Could you check a few things on this drawing? It's one solid part, dimensions in mm from its lowest x, y, z. A direction names the side the tool comes from. Give positions to 0.01 mm unless a question says otherwise; leave off trailing zeros. Order: outer loops, then holes, each group sorted by start corner. A loop starts at its lowest first (then second) coordinate and runs counter-clockwise, first axis right, second up.
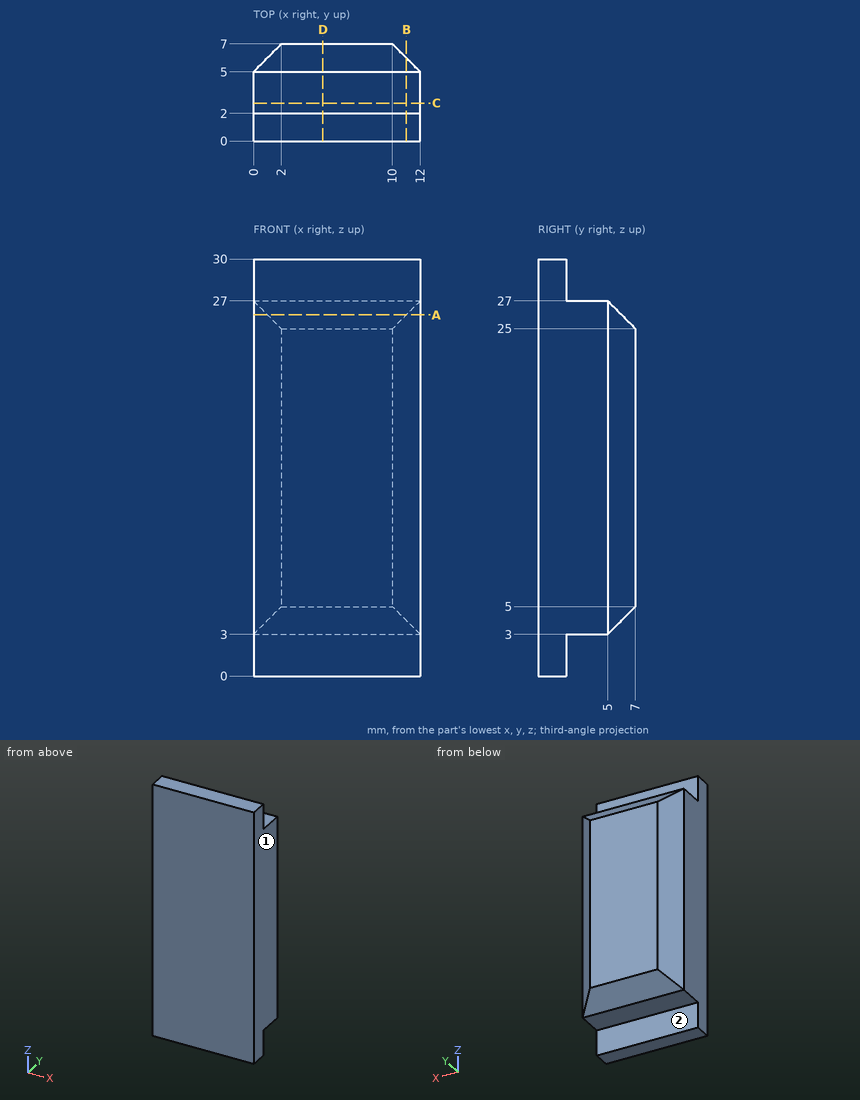
Item 1: Imagine slicing it at C-C on y = 2.75. List the corners of the cut face in (x, z) for me, then the cut area to 3 significant figures.
Findings:
outline: (0, 3) - (12, 3) - (12, 27) - (0, 27) - close
area: 288 mm2
Item 2: Imagine slicing it at D-D on x = 5. List the corners of the cut face in (y, z) for me.
Findings:
outline: (0, 0) - (2, 0) - (2, 3) - (5, 3) - (7, 5) - (7, 25) - (5, 27) - (2, 27) - (2, 30) - (0, 30) - close
Item 3: For the marked faces 1 and 2, which set-ups out of +Z, -Z, +X, -X, +Y, -Y let a thin tool reach every point of the face, with its end or its side?
Findings:
face 1: +Z, -Z, +X, +Y, -Y
face 2: -Z, +X, -X, +Y
Item 4: Imagine slicing it at B-B on x = 11. List the corners of the cut face in (y, z) for me.
Findings:
outline: (0, 0) - (2, 0) - (2, 3) - (5, 3) - (6, 4) - (6, 26) - (5, 27) - (2, 27) - (2, 30) - (0, 30) - close
Item 5: Imagine slicing it at A-A on z = 26. List the corners of the cut face in (x, y) for me.
Findings:
outline: (0, 0) - (12, 0) - (12, 5) - (11, 6) - (1, 6) - (0, 5) - close
Item 6: Please list where these lines run through material, in increasing order: line 1 along Z through (x, y) = (3, 3); line 2 along Y through (x, z) = (4.25, 28.5); line 3 along Z through (x, y) = (7.75, 6).
Findings:
line 1: z = 3 to 27
line 2: y = 0 to 2
line 3: z = 4 to 26
Item 7: For pin 1 (1.5 mm diameter, centred on x = 5, y = 3.5, fed in from +Z); pin 2 (1 mm diameter, centred on x = 2, y = 3.5, fed in from -Z); pin 3 (4 mm diameter, centred on x = 4, y = 3, fed in from -Z); pin 4 (0.9 mm diameter, centred on x = 7, z = 2, fed in from +Y), each with a flat end and sliding along its axis, tell me the tip position at first contact or that it passes through.
Findings:
pin 1: stops at z = 27
pin 2: stops at z = 3
pin 3: stops at z = 0
pin 4: stops at y = 2
